from build123d import *

# Parameters (mm, degrees)
SKETCH1_W           = 50
SKETCH1_H           = 30
BOSS_EXTRUDE1_DEPTH = 15
SKETCH2_R           = 4
BOSS_EXTRUDE2_DEPTH = 10
SKETCH3_R           = 7.5
BOSS_EXTRUDE3_DEPTH = 2
FILLET1_R           = 2


with BuildPart() as part:
    # Sketch1 → Boss-Extrude1 (new body)
    with BuildSketch(Plane.XY):
        Rectangle(SKETCH1_W, SKETCH1_H)
    extrude(amount=BOSS_EXTRUDE1_DEPTH)

    # Sketch2 → Boss-Extrude2 (add)
    with BuildSketch(Plane(origin=(0, 0, 0), x_dir=(-1, 0, 0), z_dir=(0, 0, -1))):
        with Locations((-18, 0)):
            Circle(SKETCH2_R)
        with Locations((18, 0)):
            Circle(SKETCH2_R)
    extrude(amount=BOSS_EXTRUDE2_DEPTH)

    # Sketch3 → Boss-Extrude3 (add)
    with BuildSketch(Plane.XY.offset(15)):
        Circle(SKETCH3_R)
    extrude(amount=BOSS_EXTRUDE3_DEPTH)

    # Fillet1
    fillet1_edges = [part.edges().sort_by_distance(p)[0] for p in [
        (-7.5, 0, 17),
    ]]
    fillet(fillet1_edges, radius=FILLET1_R - 0.0001)  # a hair under: the kernel refuses the full size


solid = part.part
Work out the finished part from the listing and answer in its coordinate system (mm). A direction names the side the tool comes from. Coordinates: 2 decimals unless noted, no trailing zeros. Loops run counter-clockwise (first coordinate to the right, second up) from the corner with the lowest first, then second, coordinate; pieces in that order, holes last. Notation, with made-up numbers: (-4, -18) -> (20, -18) arc R22 ccw to (20, 14) -> close; hole circle Ø9 at (34, 80). An arc over 180 degrees is marked (long way). Answer as CSV lines item,"result".
1) Straight lines are drawn through the part: probe 1 along Z at (x, y) = (-11.5, -4.5); probe 2 along Z at (x, y) = (-18, 3.5); probe 3 along X at (y, z) = (-1.75, -8.5). For each, find the intervals that lie inside material, in ascending order.
A:
probe 1,"z = 0 to 15"
probe 2,"z = -10 to 15"
probe 3,"x = -21.6 to -14.4, 14.4 to 21.6"
2) For faces 1 (the face through (-18, 0, -10)), 2 (the face through (-14, 0, -5)), determine the directions among +Z, -Z, +X, -X, +Y, -Y from which every point of the face is accessible in a straight line to the end or side of a thin tool.
A:
face 1,"-Z, +X, -X, +Y, -Y"
face 2,"-Z"
3) The part is cut by section B-B (z = -4.25). Give the vertices of the cut face in (x, y).
A:
outline,"circle Ø8 at (-18, 0); circle Ø8 at (18, 0)"
4) A flat-ended cylindrical pin translates along its axis: pin 1 (10 mm diameter, centred on x = -13, y = -9.5, fed in from +Z). Find the tip coordinate at first contact, or state that the pin passes through.
A:
pin 1,"stops at z = 15"
5) For a pull along X with two mould halves and no side action, classify faces 3 (the face through (25, 0, 7)), 4 (the face through (0, 0, 0)), 5 (the face through (0, 15, 7)) as released by +X, released by -X, zero draft, split by the parting line, or undercut.
A:
face 3,"released by +X"
face 4,"undercut"
face 5,"zero draft"
6) The part is cut by section A-A (x = 18). Give the vertices of the cut face in (y, z).
A:
outline,"(-15, 0) -> (-4, 0) -> (-4, -10) -> (4, -10) -> (4, 0) -> (15, 0) -> (15, 15) -> (-15, 15) -> close"
